Autodesk Inventor part; units mm, degrees
ref_plane "YZ Plane" through (0, 0, 0) normal (1, 0, 0) x (0, 1, 0)
ref_plane "XZ Plane" through (0, 0, 0) normal (0, 1, 0) x (-1, 0, 0)
ref_plane "XY Plane" through (0, 0, 0) normal (0, 0, 1) x (1, 0, 0)
sketch "Sketch1" plane through (0, 0, 0) normal (0, 1, 0) x (-1, 0, 0)
  line L0 (0, 0) -> (40, 0)
  line L1 (40, 0) -> (40, 40)
  line L2 (40, 40) -> (0, 40)
  line L3 (0, 40) -> (0, 0)
  dimension "d0" = 40
  dimension "d1" = 40
extrude "Extrusion1" add sketch "Sketch1" along normal blind 20
sketch "Sketch2" plane through (0, 20, 0) normal (0, 1, 0) x (1, 0, 0)
  line L0 (0, -40) -> (0, 0)
  line L1 (-40, 0) -> (-40, -40)
  line L2 (0, 0) -> (-40, 0)
  line L3 (-40, 0) -> (-40, -15)
  line L4 (-40, -15) -> (0, -15)
  line L5 (0, -15) -> (0, 0)
  dimension "d4" = 15
extrude "Extrusion2" add sketch "Sketch2" along normal blind 20
sketch "Sketch3" plane through (-40, 20, 15) normal (0, 0, 1) x (1, 0, 0)
  circle A0 centre (19.125, 9.6739) radius 5
  point P0 (40, -20)
  dimension "d7" = 10
extrude "Extrusion3" cut sketch "Sketch3" against normal blind 20
sketch "Sketch4" plane through (-40, 20, 15) normal (0, 0, 1) x (1, 0, 0)
  line L0 (40, 20) -> (0, 20)
  line L1 (40, -20) -> (40, 20)
  line L2 (0, 20) -> (40, 20)
  line L3 (40, 20) -> (40, 10)
  line L4 (40, 10) -> (0, 10)
  line L5 (0, 10) -> (0, 20)
  dimension "d10" = 10
extrude "Extrusion4" cut sketch "Sketch4" against normal blind 20
fillet "Fillet1" radius 2 4 edges at (-40, 30, 7.5) (-25.8644, 30, 7.5) (-15.8857, 30, 7.5) (0, 30, 7.5)
sketch "Sketch5" plane through (0, 20, 0) normal (0, 1, 0) x (1, 0, 0)
  line L0 (-4.8773, 1.27) -> (4.8773, 1.27) construction
  line L1 (4.8773, 1.27) -> (4.8773, -1.27) construction
  line L2 (4.8773, -1.27) -> (-4.8773, -1.27) construction
  line L3 (-4.8773, -1.27) -> (-4.8773, 1.27) construction
  point P0 (0, 0)
equation "\"BendRadius\" = Thickness"
equation "\"BendReliefWidth\" = Thickness"
equation "\"BendReliefDepth\" = 0.5 * Thickness"
equation "\"CornerReliefSize\" = 4 * Thickness"
equation "\"MinimumRemnant\" = 2 * Thickness"
equation "\"TransitionRadius\" = BendRadius"
equation "\"JacobiRadiusSize\" = BendRadius"
equation "\"GapSize\" = Thickness"
properties part number "DIODA"
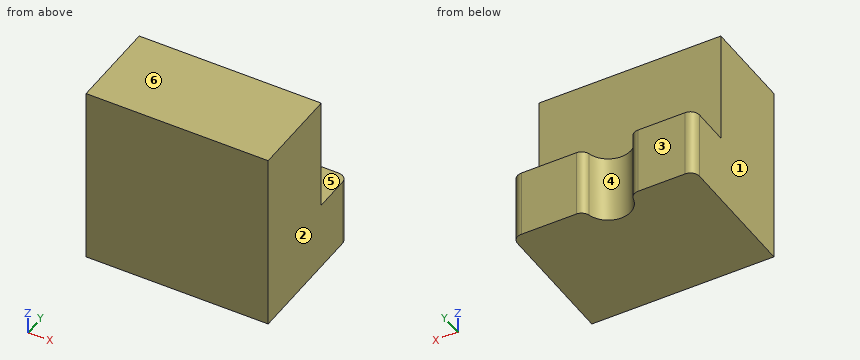
The listing builds one solid part. Answer for the finished solid, in the listing's coordinates (mm). Face numbers are marked on the shaded views. A direction names the side the tool comes from. Round coordinates to 2 decimals unless told otherwise and drop trailing zeros. Loops run counter-clockwise (first coordinate to the right, second up) from the corner with the lowest first, then second, coordinate; pieces in that order, holes last. Notation, with made-up numbers: (12, 84.5) -> (65, 84.5) arc R22 cw to (65, 118.5) -> close; hole circle Ø5 at (-30.75, 4.25). An arc over 180 degrees is marked (long way). Use one line per item in the form item = value.
1. The part is cut by section D-D on y = 23. Determine the outline of the cut face in (x, z), and give its area (3 significant figures).
Answer key:
outline = (-40, 0) -> (0, 0) -> (0, 15) -> (-40, 15) -> close
area = 600 mm²
2. For a pull along X with two mould halves and no side action, classify the marked faces 1, 2, 3 and 4 as released by +X, released by -X, zero draft, split by the parting line, or undercut.
Answer key:
face_1 = released by -X
face_2 = released by +X
face_3 = zero draft
face_4 = undercut
3. The part is cut by section B-B on z = 13.5. Determine the outline of the cut face in (x, y) (3 decimals).
Answer key:
outline = (-40, 0) -> (0, 0) -> (0, 28) arc R2 ccw to (-2, 30) -> (-14.078, 30) arc R2 ccw to (-16.02, 28.478) arc R5 cw to (-25.73, 28.478) arc R2 ccw to (-27.672, 30) -> (-38, 30) arc R2 ccw to (-40, 28) -> close
4. The part is cut by section A-A on y = 27.25. Determine the outline of the cut face in (x, z).
Answer key:
outline = (-40, 0) -> (-25.25, 0) -> (-25.25, 15) -> (-40, 15) -> close; (-16.5, 0) -> (0, 0) -> (0, 15) -> (-16.5, 15) -> close
5. A tool of negligible diameter and unlimited length cuts with its end or side. For the marked faces 5 and 6, from which of +Z, -Z, +X, -X, +Y, -Y can it reach the whole face along a straight path? Write none if from no direction.
Answer key:
face_5 = +Z, +X, -X, +Y
face_6 = +Z, +X, -X, +Y, -Y
6. A flat-ended cylindrical pin translates along its axis: pin 1 Ø4 at (y, z) = (20, 30) entering from +X. Find the tip coordinate at first contact, or state that the pin passes through.
Answer key:
pin_1 = 0
7. The part is cut by section C-C on x = -9. Determine the outline of the cut face in (y, z).
Answer key:
outline = (0, 0) -> (30, 0) -> (30, 15) -> (20, 15) -> (20, 40) -> (0, 40) -> close
8. Find the intervals of material crossed by probe 1 along Z at (x, y) = (-7, 26); probe 2 along Y at (x, z) = (-14.5, 31); probe 3 along Y at (x, z) = (-20.5, 6), in increasing order. Write a range as [from, to].
Answer key:
probe_1 = [0, 15]
probe_2 = [0, 20]
probe_3 = [0, 24.69]
